Verification items for the finished model (mm, model axes). A direction names the side the tool comes from. Round coordinates to 2 decimals unless told otherwise and drop trailing zeros. Write each loop counter-clockwise with the first axis right and the second up, starting at its lowest first coordinate (ties: lowest second). Pieces come first, ordered by that corner, then holes. Notation, with made-up numbers: M 30.25,47.25 L 56.25,47.25 A27 ccw 56.25,74.25 Z; hole C 20.5,-36 d4. An arc over 180 degrees is marked long. Use a Markdown table: item, result. Add a question column.
from build123d import *

# Parameters (mm, degrees)
EXTRUDE_1_DEPTH     = 3
SKETCH_2_R          = 2.5
CUT_EXTRUDE_1_DEPTH = 82.449370777


with BuildPart() as part:
    # 草图1 → 凸台-拉伸1 (new body)
    with BuildSketch(Plane.XY):
        with BuildLine():
            Line((-12, 0), (12, 0))
            ThreePointArc((12, 0), (14.121320344, 0.878679656), (15, 3))
            Line((15, 3), (15, 77))
            ThreePointArc((15, 77), (14.121320344, 79.121320344), (12, 80))
            Line((12, 80), (-12, 80))
            ThreePointArc((-12, 80), (-14.121320344, 79.121320344), (-15, 77))
            Line((-15, 77), (-15, 3))
            ThreePointArc((-15, 3), (-14.121320344, 0.878679656), (-12, 0))
        make_face()
    extrude(amount=EXTRUDE_1_DEPTH)

    # 草图2 → 切除-拉伸1 (cut, through all)
    with BuildSketch(Plane.XY):
        with Locations((0, 8)):
            Circle(SKETCH_2_R)
        with Locations((0, 72)):
            Circle(SKETCH_2_R)
        with BuildLine():
            Line((-5, 35), (5, 35))
            ThreePointArc((5, 35), (10, 40), (5, 45))
            Line((5, 45), (-5, 45))
            ThreePointArc((-5, 45), (-10, 40), (-5, 35))
        make_face()
    extrude(amount=CUT_EXTRUDE_1_DEPTH, mode=Mode.SUBTRACT)


solid = part.part
1. Scan lines: line 1 along X through (y, z) = (8, 0.8); line 2 along Y through (x, z) = (0, 1.1); line 3 along Y through (x, z) = (7, 1.9). Record each from-to range of solid material in increasing order. Write a range as from..to.
2. Cross-section at C-C on z = 1.4. Enter the section's corners in (x, y), plus the area to 3 significant figures.
3. Depth check by flat-ended pin: pin 1 Ø8 at (x, y) = (-3, 15.5) entering from -Z; pin 2 Ø3 at (x, y) = (0, 8) entering from +Z. Enter the tip coordinate at first touch or a pass-through.
4. Access from +Z, -Z, +X, -X, +Y, -Y to the whole of each face (thin tool, end or side, straight path). Record for faces 5 (the cylindrical face through (-10, 40, 1)), 6 (the flat face through (0, 0, 1)).
5. Cross-section at A-A on x = 8. Enter the section's corners in (y, z), plus the area to 3 significant figures.
6. Release check for a two-part mould opening along X. For faces 1 (the flat face through (-15, 41, 1)), 2 (the flat face through (0, 35, 1)), 3 (the flat face through (0, 45, 1)), 4 (the cylindrical face through (14.14, 79.1, 1.48)) record: +X half, -X half, draft (parallel to the pull), parting line (faces both ways), or undercut.
7. Cross-section at B-B on y = 72. Enter the section's corners in (x, z), plus the area to 3 significant figures.
8. Cross-section at D-D on x = 0. Enter the section's corners in (y, z), plus the area to 3 significant figures.
Answer:
| question | item | result |
|---|---|---|
| 1 | line 1 | x = -15..-2.5, 2.5..15 |
| 1 | line 2 | y = 0..5.5, 10.5..35, 45..69.5, 74.5..80 |
| 1 | line 3 | y = 0..35.42, 44.58..80 |
| 2 | outline | M -15,3 A3 ccw -12,0 L 12,0 A3 ccw 15,3 L 15,77 A3 ccw 12,80 L -12,80 A3 ccw -15,77 Z; hole M -5,35 L 5,35 A5 ccw 5,45 L -5,45 A5 ccw Z; hole C 0,8 d5; hole C 0,72 d5 |
| 2 | area | 2,170 mm^2 |
| 3 | pin 1 | stops at z = 0 |
| 3 | pin 2 | passes through |
| 4 | face 5 | +Z, -Z |
| 4 | face 6 | +Z, -Z, +X, -X, -Y |
| 5 | outline | M 0,0 L 36,0 L 36,3 L 0,3 Z; M 44,0 L 80,0 L 80,3 L 44,3 Z |
| 5 | area | 216 mm^2 |
| 6 | face 1 | -X half |
| 6 | face 2 | undercut |
| 6 | face 3 | undercut |
| 6 | face 4 | +X half |
| 7 | outline | M -15,0 L -2.5,0 L -2.5,3 L -15,3 Z; M 2.5,0 L 15,0 L 15,3 L 2.5,3 Z |
| 7 | area | 75.0 mm^2 |
| 8 | outline | M 0,0 L 5.5,0 L 5.5,3 L 0,3 Z; M 10.5,0 L 35,0 L 35,3 L 10.5,3 Z; M 45,0 L 69.5,0 L 69.5,3 L 45,3 Z; M 74.5,0 L 80,0 L 80,3 L 74.5,3 Z |
| 8 | area | 180 mm^2 |
